For this review, take the finished solid that the model builds, in its own axes (mm). A direction names the side the tool comes from. Round coordinates to 2 decimals unless told otherwise and drop trailing zeros. Write each loop counter-clockwise with the first axis right and the second up, starting at its lowest first coordinate (ties: lowest second). Pieces come first, ordered by that corner, then holes.
from build123d import *

# Parameters (mm, degrees)
SKETCH_1_R      = 1.6
EXTRUDE_1_DEPTH = 2
SKETCH_2_R      = 5
EXTRUDE_2_DEPTH = 7.7
SKETCH_3_R      = 6.5
SKETCH_3_R_2    = 5
EXTRUDE_3_DEPTH = 19.5
SKETCH_4_R      = 4
SKETCH_5_R      = 1
EXTRUDE_4_DEPTH = 11


with BuildPart() as part:
    # 草图1 → 凸台-拉伸1 (new body)
    with BuildSketch(Plane.XY):
        with BuildLine():
            Line((0.933236487, 5.304565516), (-7.256880734, 5.304565516))
            Line((-7.256880734, 5.304565516), (-13.994027653, 3.137664263))
            ThreePointArc((-13.994027653, 3.137664263), (-16.256880734, -0.465434484), (-13.994027653, -4.068533231))
            Line((-13.994027653, -4.068533231), (-7.256880734, -6.235434484))
            Line((-7.256880734, -6.235434484), (0.743119266, -6.235434484))
            Line((0.743119266, -6.235434484), (7.344389981, -4.130940192))
            ThreePointArc((7.344389981, -4.130940192), (9.743119266, -0.465434484), (7.344389981, 3.200071224))
            Line((7.344389981, 3.200071224), (0.933236487, 5.304565516))
        make_face()
        with Locations((-12.256880734, -0.465434484)):
            Circle(SKETCH_1_R, mode=Mode.SUBTRACT)
        with Locations((5.743119266, -0.465434484)):
            Circle(SKETCH_1_R, mode=Mode.SUBTRACT)
    extrude(amount=EXTRUDE_1_DEPTH)

    # 草图2 → 凸台-拉伸2 (add)
    with BuildSketch(Plane(origin=(0, 0, 0), x_dir=(-1, 0, 0), z_dir=(0, 0, -1))):
        with Locations((3.256880734, -0.465434484)):
            Circle(SKETCH_2_R)
    extrude(amount=EXTRUDE_2_DEPTH)

    # 草图3 → 凸台-拉伸3 (add)
    with BuildSketch(Plane(origin=(0, 0, -7.7), x_dir=(-1, 0, 0), z_dir=(0, 0, -1))):
        with Locations((3.256880734, -0.465434484)):
            Circle(SKETCH_3_R)
        with Locations((3.256880734, -0.465434484)):
            Circle(SKETCH_3_R_2, mode=Mode.SUBTRACT)
        with BuildLine():
            ThreePointArc((-1.743119266, -0.465434484), (3.256880734, -5.465434484), (8.256880734, -0.465434484))
            Line((8.256880734, -0.465434484), (-1.743119266, -0.465434484))
        make_face()
        with BuildLine():
            Line((-1.743119266, -0.465434484), (8.256880734, -0.465434484))
            ThreePointArc((8.256880734, -0.465434484), (3.256880734, 4.534565516), (-1.743119266, -0.465434484))
        make_face()
    extrude(amount=EXTRUDE_3_DEPTH)

    # 草图4 → section 0 of loft_1
    with BuildSketch(Plane(origin=(0, 0, -32.7), x_dir=(-1, 0, 0), z_dir=(0, 0, -1)), mode=Mode.PRIVATE) as loft_1_s0:
        with Locations((3.256880734, -0.465434484)):
            Circle(SKETCH_4_R)
    # loft up to a face of the part (loft_1)
    loft([loft_1_s0.sketch, part.faces().sort_by_distance((-3.256880734, -0.465434484, -27.2))[0]])

    # 草图5 → 凸台-拉伸4 (add)
    with BuildSketch(Plane(origin=(0, 0, -32.7), x_dir=(-1, 0, 0), z_dir=(0, 0, -1))):
        with Locations((3.256880734, -0.465434484)):
            Circle(SKETCH_5_R)
    extrude(amount=EXTRUDE_4_DEPTH)


solid = part.part
(1) We need section B-B, the plane z = -33.5. Give the boundary of the cut face in (x, y).
Geometry check:
outline: circle Ø2 at (-3.26, -0.47)
(2) Mouldability with a two-part tool opening along X and no side actions: class faces 1 (the face through (-13.855, -0.395, 0.986)), 2 (the face through (-10.578, 4.236, 0.986)), 3 (the face through (-3, 5.305, 1)), 4 (the face through (5.4, -2.03, 0.99)) as pulls with the +X half, pulls with the -X half, needs draft (parallel to the pull), parting line crosses it, or undercut.
Geometry check:
face 1: undercut
face 2: pulls with the -X half
face 3: needs draft
face 4: undercut
(3) We need section D-D, the plane z = -20. Give the boundary of the cut face in (x, y), and give its area (3 significant figures).
Geometry check:
outline: circle Ø13 at (-3.26, -0.47)
area: 133 mm2
(4) We need section C-C, the plane x = 8.25. Give the boundary of the cut face in (y, z).
Geometry check:
outline: (-3.58, 0) - (2.65, 0) - (2.65, 2) - (-3.58, 2) - close
(5) For line 1 along Z through (x, y) = (-0.75, -0.5); line 2 along X through (y, z) = (-0.5, -5); line 3 along X through (y, z) = (-0.25, -13), list the stretches that pass through material, from the lowest coordinate up.
Geometry check:
line 1: z = -32.7 to 2
line 2: x = -8.26 to 1.74
line 3: x = -9.75 to 3.24
(6) We need section A-A, the plane x = -12.75. Give the boundary of the cut face in (y, z).
Geometry check:
outline: (-4.47, 0) - (-1.99, 0) - (-1.99, 2) - (-4.47, 2) - close; (1.06, 0) - (3.54, 0) - (3.54, 2) - (1.06, 2) - close
(7) For pin 1 Ø1 at (x, z) = (-3, -34) entering from -Y; pin 2 Ø3 at (y, z) = (0, -38.5) entering from -X; pin 3 Ø4 at (x, y) = (-10, 2) entering from -Z, all flat-tipped, find the tip position at first contact; note any pin that passes through.
Geometry check:
pin 1: stops at y = -1.47
pin 2: stops at x = -4.26
pin 3: stops at z = -30.1
(8) For faces 5 (the face through (3.998, -5.198, 0.986)), 6 (the face through (-4.1, -1.3, -32.7)), 7 (the face through (-1.3, -5.25, -7.7)), 8 (the face through (-3, -6.235, 1)), list the 3-axis set-ups (+Z, -Z, +X, -X, +Y, -Y) from which the entire face can be reached by the end or side of a thin tool; tool diameter is ignored.
Geometry check:
face 5: +Z, -Z, +X, -Y
face 6: -Z
face 7: none
face 8: +Z, +X, -X, -Y
